from build123d import *

# Parameters (mm, degrees)
SKETCH1_W           = 44.5
SKETCH1_H           = 25
BOSS_EXTRUDE1_DEPTH = 38.5
SKETCH2_W           = 41.5
SKETCH2_H           = 25
CUT_EXTRUDE1_DEPTH  = 37
FILLET1_R           = 1
SKETCH3_R           = 3
BOSS_EXTRUDE2_DEPTH = 2.5
SKETCH4_R           = 1.5
CUT_EXTRUDE2_DEPTH  = 1.5
SKETCH5_R           = 1.25
SKETCH5_R_2         = 4
CUT_EXTRUDE5_DEPTH  = 4
SKETCH6_W           = 5
SKETCH6_H           = 9.5
CUT_EXTRUDE6_DEPTH  = 44.5
SKETCH7_R           = 4
CUT_EXTRUDE7_DEPTH  = 44.5
SKETCH8_R           = 1.25
CUT_EXTRUDE8_DEPTH  = 44.5


with BuildPart() as part:
    # Sketch1 → Boss-Extrude1 (new body)
    with BuildSketch(Plane.XY):
        with Locations((22.25, 12.5)):
            Rectangle(SKETCH1_W, SKETCH1_H)
    extrude(amount=BOSS_EXTRUDE1_DEPTH)

    # Sketch2 → Cut-Extrude1 (cut)
    with BuildSketch(Plane.XY.offset(38.5)):
        with Locations((22.25, 12.5)):
            Rectangle(SKETCH2_W, SKETCH2_H)
    extrude(amount=-CUT_EXTRUDE1_DEPTH, mode=Mode.SUBTRACT)

    # Fillet1
    fillet1_edges = [part.edges().sort_by_distance(p)[0] for p in [
        (44.5, 12.5, 0),
        (0, 12.5, 0),
    ]]
    fillet(fillet1_edges, radius=FILLET1_R)

    # Sketch3 → Boss-Extrude2 (add)
    with BuildSketch(Plane.XY.offset(1.5)):
        with Locations((14.25, 4.5)):
            Circle(SKETCH3_R)
        with Locations((30.25, 4.5)):
            Circle(SKETCH3_R)
        with Locations((30.25, 20.5)):
            Circle(SKETCH3_R)
        with Locations((14.25, 20.5)):
            Circle(SKETCH3_R)
    extrude(amount=BOSS_EXTRUDE2_DEPTH)

    # Sketch4 → Cut-Extrude2 (cut)
    with BuildSketch(Plane.XY.offset(1.5)):
        with Locations((6.75, 20)):
            Circle(SKETCH4_R)
        with Locations((38.25, 20)):
            Circle(SKETCH4_R)
        with Locations((38.25, 5)):
            Circle(SKETCH4_R)
        with Locations((6.75, 5)):
            Circle(SKETCH4_R)
    extrude(amount=-CUT_EXTRUDE2_DEPTH, mode=Mode.SUBTRACT)

    # Sketch5 → Cut-Extrude5 (cut)
    with BuildSketch(Plane.XY.offset(4)):
        with Locations((22.25, 20.5)):
            Circle(SKETCH5_R)
        with Locations((30.25, 20.5)):
            Circle(SKETCH5_R)
        with Locations((14.25, 20.5)):
            Circle(SKETCH5_R)
        with Locations((22.25, 12.5)):
            Circle(SKETCH5_R_2)
        with Locations((30.25, 12.5)):
            Circle(SKETCH5_R)
        with Locations((22.25, 4.5)):
            Circle(SKETCH5_R)
        with Locations((30.25, 4.5)):
            Circle(SKETCH5_R)
        with Locations((14.25, 12.5)):
            Circle(SKETCH5_R)
        with Locations((14.25, 4.5)):
            Circle(SKETCH5_R)
    extrude(amount=-CUT_EXTRUDE5_DEPTH, mode=Mode.SUBTRACT)

    # Sketch6 → Cut-Extrude6 (cut)
    with BuildSketch(Plane(origin=(44.5, 0, 0), x_dir=(0, 0, -1), z_dir=(1, 0, 0))):
        with Locations((-6.5, 12.75)):
            Rectangle(SKETCH6_W, SKETCH6_H)
    extrude(amount=-CUT_EXTRUDE6_DEPTH, mode=Mode.SUBTRACT)

    # Sketch7 → Cut-Extrude7 (cut)
    with BuildSketch(Plane(origin=(44.5, 0, 0), x_dir=(0, 0, -1), z_dir=(1, 0, 0))):
        with Locations((-27.5, 12.5)):
            Circle(SKETCH7_R)
        with BuildLine():
            ThreePointArc((-38.5, 12.5), (-35.278174593, 20.278174593), (-27.5, 23.5))
            Line((-27.5, 23.5), (-1, 25))
            Line((-1, 25), (-38.5, 25))
            Line((-38.5, 25), (-38.5, 12.5))
        make_face()
        with BuildLine():
            ThreePointArc((-27.5, 1.5), (-35.278174593, 4.721825407), (-38.5, 12.5))
            Line((-38.5, 12.5), (-38.5, 0))
            Line((-38.5, 0), (-1, 0))
            Line((-1, 0), (-27.5, 1.5))
        make_face()
    extrude(amount=-CUT_EXTRUDE7_DEPTH, mode=Mode.SUBTRACT)

    # Sketch8 → Cut-Extrude8 (cut)
    with BuildSketch(Plane(origin=(44.5, 0, 0), x_dir=(0, 0, -1), z_dir=(1, 0, 0))):
        with Locations((-19.5, 12.5)):
            Circle(SKETCH8_R)
        with Locations((-35.5, 12.5)):
            Circle(SKETCH8_R)
        with Locations((-27.5, 4.5)):
            Circle(SKETCH8_R)
        with Locations((-12, 4.5)):
            Circle(SKETCH8_R)
        with Locations((-12, 20.5)):
            Circle(SKETCH8_R)
        with Locations((-27.5, 20.5)):
            Circle(SKETCH8_R)
    extrude(amount=-CUT_EXTRUDE8_DEPTH, mode=Mode.SUBTRACT)


solid = part.part
Here's how the part is built. I have some questions about the finished solid (model axes, mm). A direction names the side the tool comes from. Coordinates: 2 decimals unless noted, no trailing zeros. Order: outer loops, then holes, each group sorted by start corner. A loop starts at its lowest first (then second) coordinate and runs counter-clockwise, first axis right, second up. Notation, with made-up numbers: (78.25, 69.25) - (102.25, 69.25) arc R35 cw to (102.25, 104.25) - close; hole circle Ø4 at (-38, 46.25). An arc over 180 degrees is marked (long way). Use CSV: the item, a comma, the result in double quotes. Start each with the question number.
1. If we mould it in two halves opening along X, with no side actions, what happens to faces 1 (the face through (0.285, 12.675, 0.301)), 2 (the face through (1.5, 12, 16)), 3 (the face through (0.761, 20.021, 26.345))? For each: +X half, -X half, draft (parallel to the pull), parting line (faces both ways), or undercut.
2. For faces 4 (the face through (16, 21, 4)), 5 (the face through (31.405, 4.021, 2.028)), 6 (the face through (1, 17.5, 7)), which set-ups out of +Z, -Z, +X, -X, +Y, -Y let a thin tool reach every point of the face, with its end or its side?
3. I'm going to push flat-ended pins straight in: pin 1 (5 mm diameter, centred on x = 38.25, y = 20, fed in from -Z); pin 2 (2 mm diameter, centred on x = 37.5, y = 14, fed in from +Z); pin 3 (2 mm diameter, centred on y = 12.5, z = 19.5, fed in from -X); pin 4 (1.6 mm diameter, centred on x = 0.5, z = 7, fed in from +Y). Where does each tip first touch, or does it pass through?
4. Suppose I cut it at B-B on x = 22.25. List the corners of the cut face in (y, z) for me.
5. Please list where these lines run through material, in increasing order: line 1 (Y direction, x = 38.25, z = 1.1); line 2 (X direction, y = 6.75, z = 27.5); line 3 (Y direction, x = 43.6, z = 12). Write a range as from..to.
6. Suppose I cut it at C-C on z = 32.5. List the corners of the cut face in (x, y) for me, then the cut area to 3 significant figures.
7. Suppose I cut it at D-D on z = 16. List the corners of the cut face in (x, y) for me, then the cut area to 3 significant figures.
8. Suppose I cut it at A-A on x = 38.25. List the corners of the cut face in (y, z) for me, then the cut area to 3 significant figures.
Output:
1,face 1,"-X half"
1,face 2,"undercut"
1,face 3,"draft"
2,face 4,"+Z, +Y, -Y"
2,face 5,"+Z, -Z"
2,face 6,"+X, -X"
3,pin 1,"stops at z = 0"
3,pin 2,"stops at z = 1.5"
3,pin 3,"passes through"
3,pin 4,"stops at y = 24.71"
4,outline,"(0, 0) - (3.25, 0) - (3.25, 1.5) - (0.03, 1.5) - (0, 1) - close; (5.75, 0) - (8.5, 0) - (8.5, 1.5) - (5.75, 1.5) - close; (16.5, 0) - (19.25, 0) - (19.25, 1.5) - (16.5, 1.5) - close; (21.75, 0) - (25, 0) - (25, 1) - (24.97, 1.5) - (21.75, 1.5) - close"
5,line 1,"y = 0.01..3.5, 6.5..18.5, 21.5..24.99"
5,line 2,"x = 0..1.5, 43..44.5"
5,line 3,"y = 0.62..3.25, 5.75..19.25, 21.75..24.38"
6,outline,"(0, 2.7) - (1.5, 2.7) - (1.5, 22.3) - (0, 22.3) - close; (43, 2.7) - (44.5, 2.7) - (44.5, 22.3) - (43, 22.3) - close"
6,area,"58.8 mm2"
7,outline,"(0, 0.85) - (1.5, 0.85) - (1.5, 24.15) - (0, 24.15) - close; (43, 0.85) - (44.5, 0.85) - (44.5, 24.15) - (43, 24.15) - close"
7,area,"69.9 mm2"
8,outline,"(0, 0) - (3.5, 0) - (3.5, 1.5) - (0.03, 1.5) - (0, 1) - close; (6.5, 0) - (18.5, 0) - (18.5, 1.5) - (6.5, 1.5) - close; (21.5, 0) - (25, 0) - (25, 1) - (24.97, 1.5) - (21.5, 1.5) - close"
8,area,"28.5 mm2"
